from build123d import *

# Parameters (mm, degrees)
F0_W      = 18
F0_H      = 21.2
F1_DEPTH  = 40
F2_W      = 13.525
F2_H      = 2.05
F3_DEPTH  = 9.05
F4_R      = 1.732
F5_DEPTH  = 0.8
F7_W      = 18
F7_H      = 13.525
F8_DEPTH  = 30
F9_W      = 18
F9_H      = 20
F10_DEPTH = 26.475
F11_W     = 18
F11_H     = 26.475
F12_DEPTH = 21.2
F13_W     = 15
F13_H     = 14
F14_DEPTH = 35
F16_D     = 4.5
F17_W     = 7.525
F17_H     = 28.2
F18_DEPTH = 15
F19_W     = 7.525
F19_H     = 11.1
F20_DEPTH = 18.001
F21_W     = 27.05
F21_H     = 3
F22_DEPTH = 3
F23_W     = 9.05
F23_H     = 3
F24_DEPTH = 3
F25_SIZE  = 5
F26_R     = 2
F27_R     = 5


# Not quite as in the source:
# - a pattern or mirror of a feature is missing from the dataset's text; its kind, count and spacing are read off the source's solid


with BuildPart() as f1:
    # F0 (on Front) → F1 (new body)
    with BuildSketch(Plane.XZ):
        with Locations((9, -10.6)):
            Rectangle(F0_W, F0_H)
    extrude(amount=F1_DEPTH)

    # F2 (on face) → F3 (join)
    with BuildSketch(Plane.YZ.offset(18)):
        with Locations((-33.2375, -1.025)):
            Rectangle(F2_W, F2_H)
        with Locations((-33.2375, -20.175)):
            Rectangle(F2_W, F2_H)
    extrude(amount=F3_DEPTH)

    # F4 (on face) → F5 (join)
    with BuildSketch(Plane(origin=(0, 0, -2.05), x_dir=(1, 0, 0), z_dir=(0, 0, -1))):
        with Locations((22.6, 34.5260798931)):
            Circle(F4_R)
    f5 = extrude(amount=F5_DEPTH)

    # F5_copies: F5 across plane
    add(f5.mirror(Plane(origin=(0, 0, -10.6), x_dir=(-1, 0, 0), z_dir=(0, 0, -1))))

    # F7 (on face) → F8 (join)
    with BuildSketch(Plane(origin=(0, 0, -21.2), x_dir=(1, 0, 0), z_dir=(0, 0, -1))):
        with Locations((9, 33.2375)):
            Rectangle(F7_W, F7_H)
    extrude(amount=F8_DEPTH)

    # F9 (on face) → F10 (join, through all)
    with BuildSketch(Plane(origin=(0, -26.475, 0), x_dir=(-1, 0, 0), z_dir=(0, 1, 0))):
        with Locations((-9, -41.2)):
            Rectangle(F9_W, F9_H)
    extrude(amount=F10_DEPTH)

    # F11 (on face) → F12 (cut, through all)
    with BuildSketch(Plane(origin=(0, 0, -21.2), x_dir=(1, 0, 0), z_dir=(0, 0, -1))):
        with Locations((9, 13.2375)):
            Rectangle(F11_W, F11_H)
    extrude(amount=-F12_DEPTH, mode=Mode.SUBTRACT)

    # F13 (on face) → F14 (cut)
    with BuildSketch(Plane.XZ.offset(40)):
        with Locations((7.5, -41.2)):
            Rectangle(F13_W, F13_H)
    extrude(amount=-F14_DEPTH, mode=Mode.SUBTRACT)

    # F16 (through all)
    with Locations(Plane(origin=(0, 0, 0), x_dir=(-1, 0, 0), z_dir=(0, 1, 0))):
        with Locations((-10, -41.2)):
            Hole(F16_D / 2)

    # F17 (on face) → F18 (cut)
    with BuildSketch(Plane(origin=(0, 0, 0), x_dir=(0, -1, 0), z_dir=(-1, 0, 0))):
        with Locations((33.2375, -17.1)):
            Rectangle(F17_W, F17_H)
    extrude(amount=-F18_DEPTH, mode=Mode.SUBTRACT)

    # F19 (on face) → F20 (cut, through all)
    with BuildSketch(Plane.YZ.offset(18)):
        with Locations((-33.2375, -10.6)):
            Rectangle(F19_W, F19_H)
    extrude(amount=-F20_DEPTH, mode=Mode.SUBTRACT)

    # F21 (on face) → F22 (join)
    with BuildSketch(Plane.XY):
        with Locations((13.525, -38.5)):
            Rectangle(F21_W, F21_H)
        with Locations((13.525, -27.975)):
            Rectangle(F21_W, F21_H)
    extrude(amount=F22_DEPTH)

    # F23 (on face) → F24 (join)
    with BuildSketch(Plane(origin=(0, 0, -21.2), x_dir=(1, 0, 0), z_dir=(0, 0, -1))):
        with Locations((22.525, 38.5)):
            Rectangle(F23_W, F23_H)
        with Locations((22.525, 27.975)):
            Rectangle(F23_W, F23_H)
    extrude(amount=F24_DEPTH)

    # F25
    f25_edges = [f1.edges().sort_by_distance(p)[0] for p in [
        (0, -27.975, 3),
    ]]
    chamfer(f25_edges, length=F25_SIZE)

    # F26
    f26_edges = [f1.edges().sort_by_distance(p)[0] for p in [
        (0, -40, -49.7),
        (0, -40, -18.1),
        (0, -13.2375, -31.2),
        (18, -40, -37.7),
        (0, -26.475, -16.6),
    ]]
    fillet(f26_edges, radius=F26_R)

    # F27
    f27_edges = [f1.edges().sort_by_distance(p)[0] for p in [
        (5, -38.5, 3),
        (5, -27.975, 3),
    ]]
    fillet(f27_edges, radius=F27_R)


solid = f1.part
Can you work these out from the model? Positions are in its coordinate system, mm. A direction names the side the tool comes from. Give positions to 0.01 mm unless a question says otherwise; leave off trailing zeros. Loops run counter-clockwise (first coordinate to the right, second up) from the corner with the lowest first, then second, coordinate; pieces in that order, holes last. Notation, with made-up numbers: (1, 20.25) -> (19, 20.25) arc R12 ccw to (19, 31.25) -> close; hole circle Ø1 at (-4, 85). An arc over 180 degrees is marked (long way). Return JSON: item names as keys, results as strings.
Q1. I want a section at D-D, the plane x = 22.6. List the corners of the cut face in (y, z) for me (3 decimals).
Checks:
{"outline": "(-40, -24.2) -> (-37, -24.2) -> (-37, -21.2) -> (-29.475, -21.2) -> (-29.475, -24.2) -> (-26.475, -24.2) -> (-26.475, -19.15) -> (-32.794, -19.15) -> (-32.794, -18.35) -> (-36.258, -18.35) -> (-36.258, -19.15) -> (-40, -19.15) -> close; (-40, -2.05) -> (-36.258, -2.05) -> (-36.258, -2.85) -> (-32.794, -2.85) -> (-32.794, -2.05) -> (-26.475, -2.05) -> (-26.475, 3) -> (-29.475, 3) -> (-29.475, 0) -> (-37, 0) -> (-37, 3) -> (-40, 3) -> close"}
Q2. For pin 1 Ø2.5 at (x, y) = (23, -35) entering from +Z; pin 2 Ø4 at (x, z) = (9.5, -43) entering from -Y; pin 3 Ø5 at (y, z) = (-35, -33) entering from +X, each with a flat end and sliding along its axis, tell me the tip position at first contact or that it passes through.
Checks:
{"pin 1": "stops at z = 0", "pin 2": "stops at y = -5", "pin 3": "stops at x = 18"}
Q3. I want a section at A-A, the plane x = 10. List the corners of the cut face in (y, z) for me (3 decimals).
Checks:
{"outline": "(-40, -51.2) -> (0, -51.2) -> (0, -43.45) -> (-5, -43.45) -> (-5, -48.2) -> (-40, -48.2) -> close; (-40, -34.2) -> (-5, -34.2) -> (-5, -38.95) -> (0, -38.95) -> (0, -31.2) -> (-26.475, -31.2) -> (-26.475, 3) -> (-29.475, 3) -> (-29.475, 0) -> (-37, 0) -> (-37, 3) -> (-40, 3) -> close; hole (-37, -31.2) -> (-29.475, -31.2) -> (-29.475, -3) -> (-37, -3) -> close"}
Q4. I need wall thicknesses on probe 1 along Z at (x, y) = (10, -2.45); probe 2 along Y at (x, z) = (16.25, -14) (3 decimals); probe 3 along Z at (x, y) = (6.5, -25). Which ranges of each line are inside material? Lowest first, please.
Checks:
{"probe 1": "z = -51.2 to -43.45, -38.95 to -31.2", "probe 2": "y = -40 to -37, -29.475 to -26.475", "probe 3": "z = -51.2 to -48.2, -34.2 to -31.2"}
Q5. We'd pull the mould along Z, two halves only. Please class faces 6 (the face through (23, -35, -2.85)), 7 (the face through (17, -28, 3)), 8 (the face through (0.6, -39.43, -16.86)): released by +Z, released by -Z, zero draft, split by the parting line, or undercut.
Checks:
{"face 6": "undercut", "face 7": "released by +Z", "face 8": "zero draft"}
Q6. I want a section at C-C, the plane y = -3. List the corners of the cut face in (x, z) for me.
Checks:
{"outline": "(0, -51.2) -> (18, -51.2) -> (18, -31.2) -> (2, -31.2) arc R2 ccw to (0, -33.2) -> close; hole circle Ø4.5 at (10, -41.2)"}
Q7. I want a section at B-B, the plane z = -41.2. List the corners of the cut face in (x, y) for me.
Checks:
{"outline": "(0, -5) -> (7.75, -5) -> (7.75, 0) -> (0, 0) -> close; (12.25, -5) -> (15, -5) -> (15, -40) -> (16, -40) arc R2 ccw to (18, -38) -> (18, 0) -> (12.25, 0) -> close"}
Q8. On a 3-axis mill with a long thin cutter (end or side, diameter ignored), from which of +Z, -Z, +X, -X, +Y, -Y can I reach the whole of each face in a straight line? I mean faces 1 (the face through (10, -13, -31.2)), 2 (the face through (22, -33, -21.2)), 3 (the face through (15, -33, -24)), 4 (the face through (14, -37, 1)), 5 (the face through (22.225, -32.835, -2.444)). Say none if no direction works.
Checks:
{"face 1": "+Z, +X, -X, +Y", "face 2": "-Z, +X", "face 3": "-X", "face 4": "+Z, +X, -X", "face 5": "none"}
